Source: CAD feature listing. Evaluate the final solid. Frame: model axes, mm. Round coordinates to 2 decimals unless told otherwise and drop trailing zeros. Write each loop counter-clockwise with the first axis right and the second up, starting at its lowest first coordinate (ties: lowest second). Pieces come first, ordered by that corner, then holes. Notation, with made-up numbers: M -5.5,-3 L 16.5,-3 A21 ccw 16.5,4 Z; hole C 51,79 d9. An arc over 180 degrees is marked long. Use a Markdown table: item, result.
```python
from build123d import *

# Parameters (mm, degrees)
SKETCH1_R               = 2.38125
BOSS_EXTRUDE1_DEPTH     = 43
SKETCH2_R               = 1.190625
CUT_EXTRUDE1_DEPTH      = 3.38125
CUT_EXTRUDE1_DEPTH_BACK = 3.38125
CHAMFER1_SIZE           = 0.5


with BuildPart() as part:
    # Sketch1 → Boss-Extrude1 (new body)
    with BuildSketch(Plane.XY):
        Circle(SKETCH1_R)
    extrude(amount=-BOSS_EXTRUDE1_DEPTH)

    # Sketch2 → Cut-Extrude1 (cut, two sides)
    with BuildSketch(Plane(origin=(0, 0, 0), x_dir=(1, 0, 0), z_dir=(0, 1, 0))) as cut_extrude1_sk:
        with Locations((0, 6.75)):
            Circle(SKETCH2_R)
    extrude(amount=CUT_EXTRUDE1_DEPTH, mode=Mode.SUBTRACT)
    extrude(cut_extrude1_sk.sketch, amount=-CUT_EXTRUDE1_DEPTH_BACK, mode=Mode.SUBTRACT)

    # Chamfer1
    chamfer1_edges = [part.edges().sort_by_distance(p)[0] for p in [
        (-2.38125, 0, 0),
        (-2.38125, 0, -43),
    ]]
    chamfer(chamfer1_edges, length=CHAMFER1_SIZE)


solid = part.part
```
Q1. Section C-C on z = -6. Return loops of the section in (x, y), plus the area to 3 significant figures.
Results are:
| item | result |
|---|---|
| outline | M -0.92,-2.19 L -0.92,2.19 A2.38 ccw Z; M 0.92,-2.19 A2.38 ccw 0.92,2.19 Z |
| area | 9.23 mm^2 |
Q2. First-contact query: pin 1 Ø1.5 at (x, z) = (2, -12) entering from -Y; pin 2 Ø1.4 at (x, z) = (0, -6.75) entering from +Y; pin 3 Ø1.5 at (y, z) = (1.5, -23.5) entering from -X. Flat tips, straight axial feed; report the tip coordinate or a pass-through.
Results are:
| item | result |
|---|---|
| pin 1 | y = -2.03 |
| pin 2 | through |
| pin 3 | x = -2.26 |
Q3. Section B-B on z = -13. Return loops of the section in (x, y).
Results are:
| item | result |
|---|---|
| outline | C 0,0 d4.76 |
Q4. Line query: L1, parallel to Z at x = 0, y = -1.4; L2, parallel to Z at x = 0.75, y = 1.1; L3, parallel to Y at x = -0.1, z = -3.5. Output: solid intervals per line, ascending.
Results are:
| item | result |
|---|---|
| L1 | -43 to -7.94, -5.56 to 0 |
| L2 | -43 to -7.67, -5.83 to 0 |
| L3 | -2.38 to 2.38 |
Q5. Section A-A on x = 0. Return loops of the section in (y, z).
Results are:
| item | result |
|---|---|
| outline | M -2.38,-42.5 L -1.88,-43 L 1.88,-43 L 2.38,-42.5 L 2.38,-7.94 L -2.38,-7.94 Z; M -2.38,-5.56 L 2.38,-5.56 L 2.38,-0.5 L 1.88,0 L -1.88,0 L -2.38,-0.5 Z |
